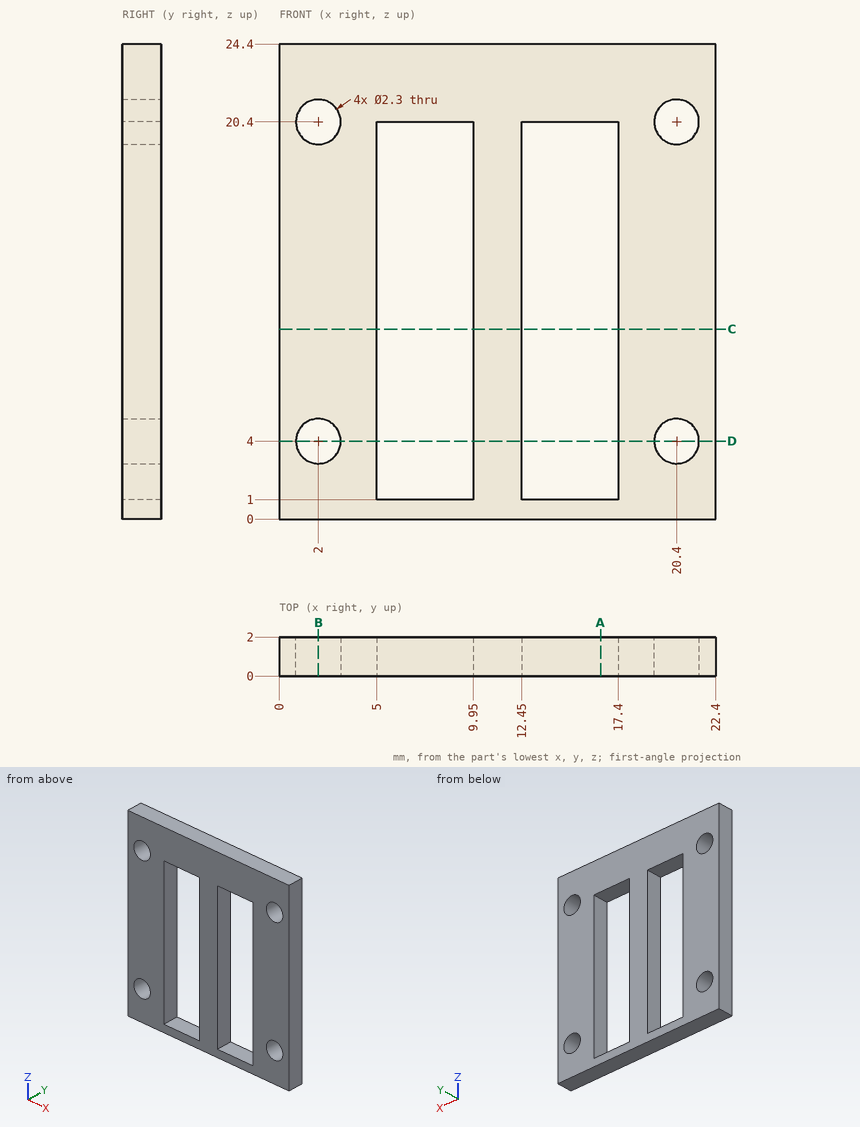
Drawing for the job (mm, zero at the part's lowest x, y, z). Round coordinates to 2 decimals unless told otherwise and drop trailing zeros. Write each loop counter-clockwise with the first axis right and the second up, starting at its lowest first coordinate (ties: lowest second). Pieces come first, ordered by that corner, then holes.
Item 1: Drill centre lines: L1, parallel to Z at x = 20.4, y = 0.95; L2, parallel to X at y = 1.75, z = 2.5. Where is each one in solid material? Low to high.
Filled in:
L1: z = 0 to 2.85, 5.15 to 19.25, 21.55 to 24.4
L2: x = 0 to 5, 9.95 to 12.45, 17.4 to 22.4
Item 2: Band-saw the part on D-D on z = 4. Write the cut outline in (x, y), then the cut area to 3 significant figures.
Filled in:
outline: (0, 0) - (0.85, 0) - (0.85, 2) - (0, 2) - close; (3.15, 0) - (5, 0) - (5, 2) - (3.15, 2) - close; (9.95, 0) - (12.45, 0) - (12.45, 2) - (9.95, 2) - close; (17.4, 0) - (19.25, 0) - (19.25, 2) - (17.4, 2) - close; (21.55, 0) - (22.4, 0) - (22.4, 2) - (21.55, 2) - close
area: 15.8 mm2
Item 3: Band-saw the part on A-A on x = 16.5. Write the cut outline in (y, z).
Filled in:
outline: (0, 0) - (2, 0) - (2, 1) - (0, 1) - close; (0, 20.4) - (2, 20.4) - (2, 24.4) - (0, 24.4) - close
Item 4: Band-saw the part on C-C on z = 9.75. Write the cut outline in (x, y), then the cut area to 3 significant figures.
Filled in:
outline: (0, 0) - (5, 0) - (5, 2) - (0, 2) - close; (9.95, 0) - (12.45, 0) - (12.45, 2) - (9.95, 2) - close; (17.4, 0) - (22.4, 0) - (22.4, 2) - (17.4, 2) - close
area: 25.0 mm2
Item 5: Band-saw the part on B-B on x = 2. Write the cut outline in (y, z), then the cut area to 3 significant figures.
Filled in:
outline: (0, 0) - (2, 0) - (2, 2.85) - (0, 2.85) - close; (0, 5.15) - (2, 5.15) - (2, 19.25) - (0, 19.25) - close; (0, 21.55) - (2, 21.55) - (2, 24.4) - (0, 24.4) - close
area: 39.6 mm2
